from build123d import *

# Parameters (mm, degrees)
SKETCH1_W           = 170
SKETCH1_H           = 85
BOSS_EXTRUDE1_DEPTH = 5
SKETCH2_W           = 5
SKETCH2_H           = 10
BOSS_EXTRUDE2_DEPTH = 10
SKETCH3_R           = 2.5
CUT_EXTRUDE1_DEPTH  = 176.87282337
SKETCH4_W           = 5
SKETCH4_H           = 25
SKETCH4_H_2         = 15
CUT_EXTRUDE2_DEPTH  = 96.557574268
CHAMFER1_SIZE       = 5


with BuildPart() as part:
    # Sketch1 → Boss-Extrude1 (new body)
    with BuildSketch(Plane(origin=(0, 0, 0), x_dir=(1, 0, 0), z_dir=(0, 1, 0))):
        Rectangle(SKETCH1_W, SKETCH1_H)
    extrude(amount=BOSS_EXTRUDE1_DEPTH)

    # Sketch2 → Boss-Extrude2 (add)
    with BuildSketch(Plane(origin=(0, 5, 0), x_dir=(1, 0, 0), z_dir=(0, 1, 0))):
        with Locations((-82.5, 12.5)):
            Rectangle(SKETCH2_W, SKETCH2_H)
        with Locations((-82.5, -12.5)):
            Rectangle(SKETCH2_W, SKETCH2_H)
        with Locations((82.5, -12.5)):
            Rectangle(SKETCH2_W, SKETCH2_H)
        with Locations((82.5, 12.5)):
            Rectangle(SKETCH2_W, SKETCH2_H)
    extrude(amount=BOSS_EXTRUDE2_DEPTH)

    # Sketch3 → Cut-Extrude1 (cut, through all)
    with BuildSketch(Plane.ZY.offset(85)):
        with Locations((-12.5, 10)):
            Circle(SKETCH3_R)
        with Locations((12.5, 10)):
            Circle(SKETCH3_R)
    extrude(amount=-CUT_EXTRUDE1_DEPTH, mode=Mode.SUBTRACT)

    # Sketch4 → Cut-Extrude2 (cut, through all)
    with BuildSketch(Plane(origin=(0, 5, 0), x_dir=(1, 0, 0), z_dir=(0, 1, 0))):
        with Locations((-82.5, 30)):
            Rectangle(SKETCH4_W, SKETCH4_H)
        with Locations((-82.5, -30)):
            Rectangle(SKETCH4_W, SKETCH4_H)
        with Locations((-82.5, 0)):
            Rectangle(SKETCH4_W, SKETCH4_H_2)
        with Locations((82.5, 0)):
            Rectangle(SKETCH4_W, SKETCH4_H_2)
        with Locations((82.5, 30)):
            Rectangle(SKETCH4_W, SKETCH4_H)
        with Locations((82.5, -30)):
            Rectangle(SKETCH4_W, SKETCH4_H)
    extrude(amount=-CUT_EXTRUDE2_DEPTH, mode=Mode.SUBTRACT)

    # Chamfer1
    chamfer1_edges = [part.edges().sort_by_distance(p)[0] for p in [
        (85, 0, 12.5),
        (85, 0, -12.5),
        (-85, 0, 12.5),
        (-85, 0, -12.5),
    ]]
    chamfer(chamfer1_edges, length=CHAMFER1_SIZE)


solid = part.part
Can you work these out from the model? Positions are in its coordinate system, mm. A direction names the side the tool comes from. Give positions to 0.01 mm unless a question says otherwise; leave off trailing zeros. Loops run counter-clockwise (first coordinate to the right, second up) from the corner with the lowest first, then second, coordinate; pieces in that order, holes last. Notation, with made-up numbers: M 9.25,-23 L 18.25,-23 A25 cw 18.25,-2 Z; hole C 13,-7 d10. An arc over 180 degrees is marked long. One line per item, written item: value. Start each with the question number.
1) If we section it at A-A, the plane y = 10: Give the number of separate pieces and of enclosed holes in the cut face, and give its area (3 significant figures).
2) If we section it at C-C, the plane y = 2.25: Write out the boundary of the cut face in (x, z), and give its area (3 significant figures).
3) I'm going to push flat-ended pins straight in: pin 1 (4 mm diameter, centred on x = -83, y = 7, fed in from -Z); pin 2 (1.5 mm diameter, centred on x = -83.5, y = 5.5, fed in from +Z); pin 3 (1.5 mm diameter, centred on y = 3.5, z = 26, fed in from -X). Where does each tip first touch, or does it pass through?
4) If I drill on line 1 (X direction, y = 6, z = 16); line 2 (Y direction, x = -5, z = -10.5); line 3 (Y direction, x = -81.05, z = -12.5), over which ranges is the centre line in solid material (lowest first)? Write a range as [from, to].
5) If we section it at D-D, the plane x = -40.5: Write out the boundary of the cut face in (y, z), and give its area (3 significant figures).
6) On a 3-axis mill with a long thin cutter (end or side, diameter ignored), from which of +Z, -Z, +X, -X, +Y, -Y can I reach the whole of each face in a straight line? I mean faces 1 (the face through (80, 9, 15)), 2 (the face through (-83, 9, -7.5)), 3 (the face through (80, 3, 30)), 4 (the face through (-83, 9, -17.5)). Say none if no direction works.
7) If we section it at B-B, the plane z = 12.5: Write out the boundary of the cut face in (x, y).
8) Thinking about a two-plate mould opening in Y: for faces 5 (the face through (82, 9, 17.5)), 6 (the face through (-83, 8, 11)), 7 (the face through (-83, 15, -13)), which applies, +Y half, -Y half, draft (parallel to the pull), parting line (faces both ways), or undercut?
Completed:
1. separate pieces: 8
1. enclosed holes: 0
1. area: 100 mm^2
2. outline: M -82.25,-17.5 L -80,-17.5 L -80,-42.5 L 80,-42.5 L 80,-17.5 L 82.25,-17.5 L 82.25,-7.5 L 80,-7.5 L 80,7.5 L 82.25,7.5 L 82.25,17.5 L 80,17.5 L 80,42.5 L -80,42.5 L -80,17.5 L -82.25,17.5 L -82.25,7.5 L -80,7.5 L -80,-7.5 L -82.25,-7.5 Z
2. area: 13,700 mm^2
3. pin 1: stops at z = -17.5
3. pin 2: stops at z = 17.5
3. pin 3: stops at x = -80
4. line 1: x = [-85, -80], [80, 85]
4. line 2: y = [0, 5]
4. line 3: y = [1.05, 7.5], [12.5, 15]
5. outline: M 0,-42.5 L 5,-42.5 L 5,42.5 L 0,42.5 Z
5. area: 425 mm^2
6. face 1: +Z, -Z, +Y
6. face 2: -X, +Y, -Y
6. face 3: +Z, +X, +Y, -Y
6. face 4: -Z, -X, +Y, -Y
7. outline: M -85,5 L -80,0 L 80,0 L 85,5 L 85,7.5 L 80,7.5 L 80,5 L -80,5 L -80,7.5 L -85,7.5 Z; M -85,12.5 L -80,12.5 L -80,15 L -85,15 Z; M 80,12.5 L 85,12.5 L 85,15 L 80,15 Z
8. face 5: draft
8. face 6: undercut
8. face 7: +Y half
